Answer from the drawing. Dimensions are ordinates in mm from the lowest x, y and z of the part. Round coordinates to 2 decimals unless told otherwise and drop trailing zeros. Write each loop counter-clockwise with the first axis right and the second up, starting at its lowest first coordinate (ties: lowest second). Pieces come first, ordered by that corner, then holes. Notation, with made-up numbers: M -4,-21 L 9,-21 A23 cw 9,-9 Z; hole C 72.25,15 d2. An arc over 180 degrees is marked long. One line per item, written item: value. Start each with the question number.
(1) Section B-B (x = 69.85) is taken. Determine the outline of the cut face in (y, z).
(2) Section A-A (z = 69.85) is taken. Determine the outline of the cut face in (x, y).
(3) Given P1, Ø1.4, axis at y = 2, z = 162.5, coming from the +X side; P2, Ø2.5, axis at y = 1.5, z = 155.5, coming from the -X side; P3, Ø1, axis at x = 109.5, y = 1, coming from the +Z side, each flat-ended and moving along its own axis, determine where each tip first touches the part or whether it passes through.
(4) Section D-D (x = 125) is taken. Determine the outline of the cut face in (y, z), plus the area to 3 significant figures.
(5) Consider probe 1 along X at (y, z) = (3.3, 69.85); probe 2 along X at (y, z) = (3.9, 144); probe 3 along Z at (x, y) = (68, 3.35) (1 decimal). Determine where each line is inside the solid, lowest interval first.
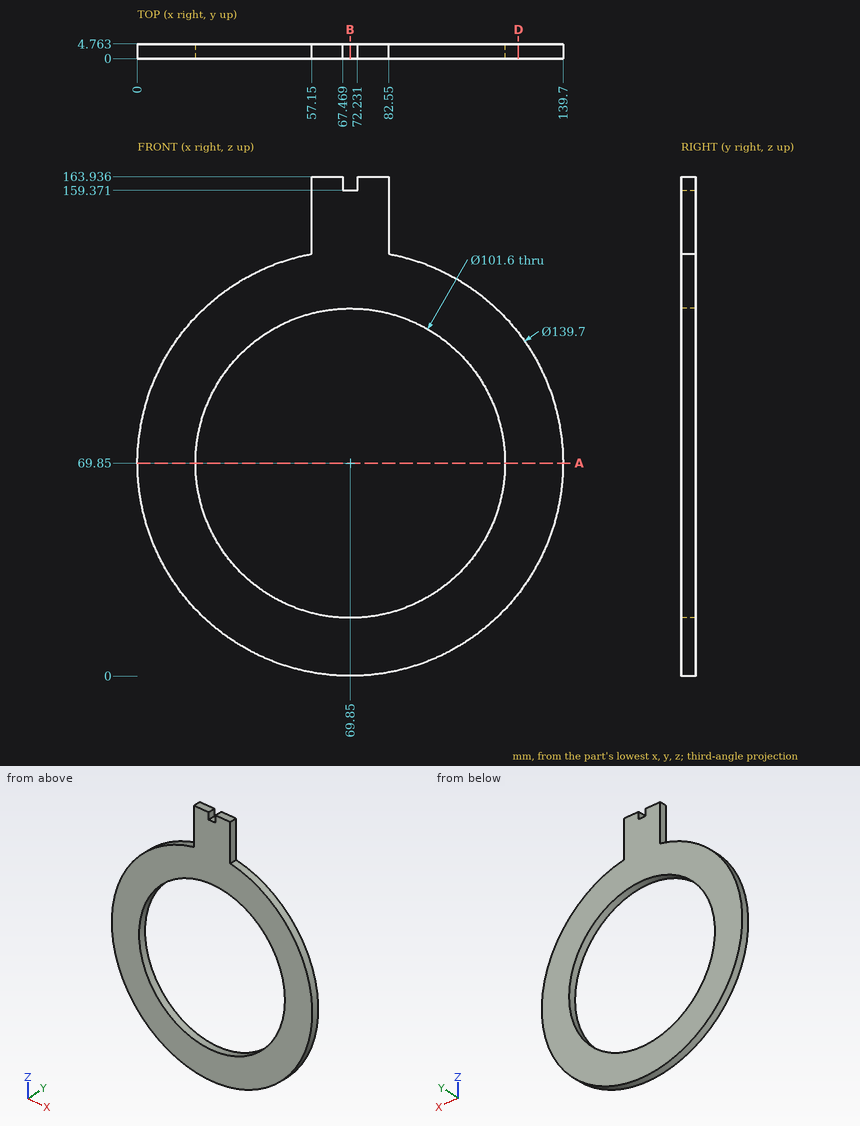
Recorded:
1. outline: M 0,0 L 4.76,0 L 4.76,19.05 L 0,19.05 Z; M 0,120.65 L 4.76,120.65 L 4.76,159.37 L 0,159.37 Z
2. outline: M 0,0 L 19.05,0 L 19.05,4.76 L 0,4.76 Z; M 120.65,0 L 139.7,0 L 139.7,4.76 L 120.65,4.76 Z
3. P1: stops at x = 82.55
3. P2: stops at x = 57.15
3. P3: stops at z = 127.7
4. outline: M 0,26.98 L 4.76,26.98 L 4.76,112.72 L 0,112.72 Z
4. area: 408 mm2
5. probe 1: x = 0 to 19.05, 120.65 to 139.7
5. probe 2: x = 57.15 to 82.55
5. probe 3: z = 0 to 19.1, 120.6 to 159.4
